from build123d import *

# Parameters (mm, degrees)
F0_W     = 25.4
F0_H     = 304.8
F1_DEPTH = 6.35
F2_R     = 2.388
F3_DEPTH = 6.351
F4_R     = 6.35
F5_DEPTH = 6.351
F6_R     = 5
F7_DEPTH = 6.351


with BuildPart() as f1:
    # F0 (on Front) → F1 (new body)
    with BuildSketch(Plane.XZ):
        with Locations((12.7, 152.4)):
            Rectangle(F0_W, F0_H)
    extrude(amount=F1_DEPTH)

    # F2 (on face) → F3 (cut, through all)
    with BuildSketch(Plane.XZ.offset(6.35)):
        with Locations((12.7, 15)):
            Circle(F2_R)
    extrude(amount=-F3_DEPTH, mode=Mode.SUBTRACT)

    # F4 (on face) → F5 (cut, through all)
    with BuildSketch(Plane.XZ.offset(6.35)):
        with Locations((12.7, 284.8)):
            Circle(F4_R)
    extrude(amount=-F5_DEPTH, mode=Mode.SUBTRACT)

    # F6 (on face) → F7 (cut, through all)
    with BuildSketch(Plane.XZ.offset(6.35)):
        with Locations((12.7, 25)):
            Circle(F6_R)
    extrude(amount=-F7_DEPTH, mode=Mode.SUBTRACT)


solid = f1.part
Input: part model. Units: mm. Frame: model coordinates. Give positions to 0.01 mm unless a question says otherwise; leave off trailing zeros. Write each loop counter-clockwise with the first axis right and the second up, starting at its lowest first coordinate (ties: lowest second). Pieces come first, ordered by that corner, then holes.
Q1. Section A-A, the plane z = 25. Output: boundary loops of the cut face in (x, y).
Q2. Section C-C, the plane z = 284.8. Output: boundary loops of the cut face in (x, y), plus the area to 3 significant figures.
Q3. Section B-B, the plane y = -4. Output: boundary loops of the cut face in (x, z), plus the area to 3 significant figures.
Q4. Material intervals for probe 1 along Z at (x, y) = (12.7, -4); probe 2 along X at (y, z) = (-2.75, 284.8), sorted ascending.
Q5. Pull-direction query (X, two-part tool) for faces 1 (the face through (25.4, -3, 150)), 2 (the face through (11.32, -3.22, 278.6)), 3 (the face through (13, -3, 0)); classes: pulls with the +X half, pulls with the -X half, needs draft (parallel to the pull), parting line crosses it, or undercut.
Q6. First-contact query: P1, Ø9, axis at x = 12.7, z = 25, coming from the -Y side. Flat tip, straight axial feed; report the tip coordinate or a pass-through.
Filled in:
1. outline: (0, -6.35) - (7.7, -6.35) - (7.7, 0) - (0, 0) - close; (17.7, -6.35) - (25.4, -6.35) - (25.4, 0) - (17.7, 0) - close
2. outline: (0, -6.35) - (6.35, -6.35) - (6.35, 0) - (0, 0) - close; (19.05, -6.35) - (25.4, -6.35) - (25.4, 0) - (19.05, 0) - close
2. area: 80.6 mm2
3. outline: (0, 0) - (25.4, 0) - (25.4, 304.8) - (0, 304.8) - close; hole circle Ø12.7 at (12.7, 284.8); hole circle Ø10 at (12.7, 25); hole circle Ø4.78 at (12.7, 15)
3. area: 7,520 mm2
4. probe 1: z = 0 to 12.61, 17.39 to 20, 30 to 278.45, 291.15 to 304.8
4. probe 2: x = 0 to 6.35, 19.05 to 25.4
5. face 1: pulls with the +X half
5. face 2: undercut
5. face 3: needs draft
6. P1: passes through
